Design review of the part built by this model. Coordinates are the model's own, in mm. Face numbers are marked on the shaded views. Round coordinates to 2 decimals unless told otherwise and drop trailing zeros. Write each loop counter-clockwise with the first axis right and the second up, starting at its lowest first coordinate (ties: lowest second). Pieces come first, ordered by that corner, then holes. Notation, with made-up numbers: M -37,60 L -14,60 A19 ccw -14,82 Z; hole C 37,23.25 d9. An arc over 180 degrees is marked long. One line per question, with ' | ' between items. Start each with the question number.
Item 1: Add section A-A, the plane z = 5. State the section outline as (x, y) points, and give its area (3 significant figures).
Item 2: Add section B-B, the plane x = -2.25. Give the number of separate pieces and of enclosed holes in the cut face, and give its area (3 significant figures).
Item 3: For L1, parallel to X at y = 0, z = 28; L2, parallel to Y at x = 0, z = 0.85, list the stretches that pass through material, from the lowest coordinate up.
Item 4: Add section C-C, the plane y = -8. State the section outline as (x, z) points, and give its area (3 significant figures).
Item 5: Draft analysis for pull direction X (two halves, no side actions). For the marked faces 1, 2 and 3, state which applies: released by +X, released by -X, zero draft, split by the parting line, or undercut.
Item 6: Insertion check: pin 1 Ø10.5 at (x, y) = (0, -1.5) entering from -Z; pin 2 Ø3 at (x, y) = (4, -7) entering from +Z; pin 3 Ø1.5 at (y, z) = (-3, 39) entering from +X; pin 4 Ø3.5 at (y, z) = (5.5, 11) entering from -X. Each pin has a flat end and moves straight along its axis. Give the tip position at first contact, or say it passes through.
Item 7: Add section D-D, the plane y = 7.75. State the section outline as (x, z) points.
Autodesk Inventor part; units mm, degrees
ref_plane "YZ Plane" through (0, 0, 0) normal (1, 0, 0) x (0, 1, 0)
ref_plane "XY Plane" through (0, 0, 0) normal (0, 0, 1) x (1, 0, 0)
sketch "Sketch1" plane through (0, 0, 0) normal (0, 0, 1) x (1, 0, 0)
  line L0 (0, 0) -> (0, 6)
  circle A0 centre (0, 6) radius 1.5
  circle A1 centre (-4.2426, 4.2426) radius 1.5
  circle A2 centre (-6, 0) radius 1.5
  circle A3 centre (-4.2426, -4.2426) radius 1.5
  circle A4 centre (0, -6) radius 1.5
  circle A5 centre (4.2426, -4.2426) radius 1.5
  circle A6 centre (6, 0) radius 1.5
  circle A7 centre (4.2426, 4.2426) radius 1.5
  circle A8 centre (0, 0) radius 9
  dimension "d0" = 6
  dimension "d1" = 3
  dimension "d4" = 360
  dimension "d6" = 18
extrude "Extrusion1" add sketch "Sketch1" along normal blind 7 contours A1 | A3 | A5 | A7 | A8
sketch "Sketch2" plane through (0, 0, 0) normal (0, 0, -1) x (-1, 0, 0)
  circle A0 centre (0, 0) radius 6.5
  dimension "d9" = 13
extrude "Extrusion2" cut sketch "Sketch2" against normal blind 1
sketch "Sketch3" plane through (0, 0, 7) normal (0, 0, 1) x (1, 0, 0)
  circle A0 centre (0, 0) radius 6.5
  dimension "d12" = 13
extrude "Extrusion3" add sketch "Sketch3" along normal blind 50
sketch "Sketch5" plane through (0, 0, 57) normal (0, 0, 1) x (1, 0, 0)
  circle A0 centre (0, 0) radius 3.25
  dimension "d25" = 6.5
extrude "Extrusion5" cut sketch "Sketch5" against normal up to surface (56 mm away)
ref_plane "Work Plane1" through (0, 12, 0) normal (0, 1, 0) x (-1, 0, 0)
sketch "Sketch8" plane through (0, 0, 7) normal (0, 0, 1) x (1, 0, 0)
  circle A0 centre (0, 0) radius 3
  dimension "d44" = 6
extrude "Extrusion8" cut sketch "Sketch8" against normal through all
sketch "Sketch9" plane through (0, 0, 0) normal (1, 0, 0) x (0, 1, 0)
  line L0 (6.5, 7) -> (6.5, 57)
  line L1 (6.5, 7) -> (6.5, 57)
  line L2 (6.3333, 7) -> (7.5, 7)
  line L3 (7.5, 7) -> (2.5, 7)
  line L4 (2.5, 7) -> (2.5, 14)
  line L5 (2.5, 14) -> (7.5, 14)
  line L6 (7.5, 14) -> (7.5, 7)
  line L7 (0, -11.4) -> (0, 68.4)
  point P0 (0, 0)
  dimension "d61" = 5
  dimension "d62" = 7
coil "Coil2" sketch "Sketch9" operation cut axis through (0, 0, 7) along (0, 0, 1) pitch 35 turns 1.428571 hand right taper 1
sketch "Boceto13" plane through (0, 0, 0) normal (0, 0, -1) x (-1, 0, 0)
  arc A0 (-6.3333, 1.4625) -> (-6.3333, -1.4625) centre (-6, 0) ccw
  circle A1 centre (-6, 0) radius 1.5
  arc A2 (-1.4625, -6.3333) -> (1.4625, -6.3333) centre (0, -6) ccw
  circle A3 centre (0, -6) radius 1.5
  arc A4 (1.4625, 6.3333) -> (-1.4625, 6.3333) centre (0, 6) ccw
  circle A5 centre (0, 6) radius 1.5
  arc A6 (6.3333, -1.4625) -> (6.3333, 1.4625) centre (6, 0) ccw
  circle A7 centre (6, 0) radius 1.5
  point P0 (0, 0)
extrude "Extrusión9" add sketch "Boceto13" against normal blind 7
sketch "Boceto14" plane through (0, 0, 1) normal (0, 0, -1) x (-1, 0, 0)
  circle A0 centre (0, 0) radius 6.5
extrude "Extrusión10" cut sketch "Boceto14" along normal blind 2
properties part number "ScrewActuatorGripper_2"
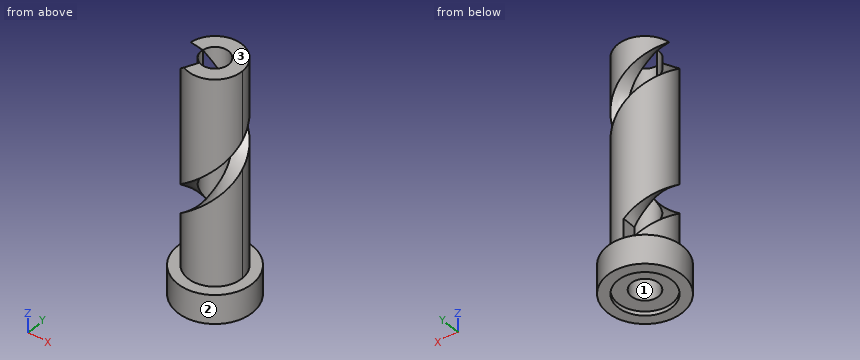
Computed values:
1) outline: C 0,0 d18; hole C 0,0 d6.5 | area: 221 mm^2
2) separate pieces: 5 | enclosed holes: 0 | area: 377 mm^2
3) L1: x = -6.5 to -3.25, 3.25 to 6.5 | L2: y = -9 to -6.5, 6.5 to 9
4) outline: M -4.12,0 L 4.12,0 L 4.12,7 L -4.12,7 Z | area: 57.7 mm^2
5) face 1: undercut | face 2: split by the parting line | face 3: zero draft
6) pin 1: stops at z = 0 | pin 2: stops at z = 7 | pin 3: stops at x = 6.1 | pin 4: stops at x = -5.31
7) outline: M -4.58,0 L 4.58,0 L 4.58,7 L -4.58,7 Z
